from build123d import *

# Parameters (mm, degrees)
SKETCH_1_R          = 1.25
SKETCH_1_R_2        = 1.5
EXTRUDE_1_DEPTH     = 2
CUT_EXTRUDE_1_DEPTH = 10
FILLET_1_R          = 2


with BuildPart() as part:
    # 草图1 → 凸台-拉伸1 (new body)
    with BuildSketch(Plane(origin=(0, 0, 0), x_dir=(1, 0, 0), z_dir=(0, 1, 0))):
        Polygon((11, 0), (-11, 0), (-16.5, -41.3), (-16.5, -120.3), (-16.5, -167.8), (23.75, -167.8), (23.75, -124.8), (16.5, -120.3), (16.5, -41.3), align=None)
        with Locations(Location((-8, -3, 0), (0, 0, 270))):
            Circle(SKETCH_1_R, mode=Mode.SUBTRACT)
        with Locations(Location((-8, -33, 0), (0, 0, 270))):
            Circle(SKETCH_1_R, mode=Mode.SUBTRACT)
        with Locations(Location((8, -33, 0), (0, 0, 90))):
            Circle(SKETCH_1_R, mode=Mode.SUBTRACT)
        with Locations(Location((8, -3, 0), (0, 0, 90))):
            Circle(SKETCH_1_R, mode=Mode.SUBTRACT)
        with Locations(Location((-13, -45.3, 0), (0, 0, 270))):
            Circle(SKETCH_1_R_2, mode=Mode.SUBTRACT)
        with Locations(Location((-13, -105.3, 0), (0, 0, 270))):
            Circle(SKETCH_1_R_2, mode=Mode.SUBTRACT)
        with Locations(Location((-13, -115.3, 0), (0, 0, 270))):
            Circle(SKETCH_1_R_2, mode=Mode.SUBTRACT)
        with Locations(Location((13, -115.3, 0), (0, 0, 90))):
            Circle(SKETCH_1_R_2, mode=Mode.SUBTRACT)
        with Locations(Location((13, -105.3, 0), (0, 0, 90))):
            Circle(SKETCH_1_R_2, mode=Mode.SUBTRACT)
        with Locations(Location((13, -45.3, 0), (0, 0, 90))):
            Circle(SKETCH_1_R_2, mode=Mode.SUBTRACT)
        with Locations(Location((20.75, -129.8, 0), (0, 0, 270))):
            Circle(SKETCH_1_R_2, mode=Mode.SUBTRACT)
        with Locations(Location((20.75, -159.8, 0), (0, 0, 90))):
            Circle(SKETCH_1_R_2, mode=Mode.SUBTRACT)
        with Locations(Location((-9.25, -164.8, 0), (0, 0, 270))):
            Circle(SKETCH_1_R_2, mode=Mode.SUBTRACT)
    extrude(amount=EXTRUDE_1_DEPTH)

    # 草图2 → 切除-拉伸1 (cut)
    with BuildSketch(Plane(origin=(0, 2, 0), x_dir=(1, 0, 0), z_dir=(0, 1, 0))):
        Polygon((6.754889433, -6), (-6.754889433, -6), (-9.951015341, -30), (9.951015341, -30), align=None)
        Polygon((12.5, -97.228932188), (2.5, -87.228932188), (2.5, -39.042640687), (12.5, -49.042640687), align=None)
        Polygon((-12.5, -49.042640687), (-2.5, -39.042640687), (-2.5, -87.228932188), (-12.5, -97.228932188), align=None)
        Polygon((-9.5, -101.3), (0, -91.8), (9.5, -101.3), (9.5, -120.3), (-9.5, -120.3), align=None)
    extrude(amount=-CUT_EXTRUDE_1_DEPTH, mode=Mode.SUBTRACT)

    # 圆角1
    fillet_1_edges = [part.edges().sort_by_distance(p)[0] for p in [
        (-9.951015341, 1, 30),
        (-6.754889433, 1, 6),
        (6.754889433, 1, 6),
        (9.951015341, 1, 30),
        (0, 1, 91.8),
        (9.5, 1, 101.3),
        (9.5, 1, 120.3),
        (-9.5, 1, 120.3),
        (-9.5, 1, 101.3),
        (12.5, 1, 49.042640687),
        (12.5, 1, 97.228932188),
        (2.5, 1, 87.228932188),
        (2.5, 1, 39.042640687),
        (-12.5, 1, 97.228932188),
        (-12.5, 1, 49.042640687),
        (-2.5, 1, 39.042640687),
        (-2.5, 1, 87.228932188),
        (23.75, 1, 124.8),
        (23.75, 1, 167.8),
        (-16.5, 1, 167.8),
        (-11, 1, 0),
        (11, 1, 0),
        (16.5, 1, 120.3),
    ]]
    fillet(fillet_1_edges, radius=FILLET_1_R)


solid = part.part
CAD build for the part. Positions are in the model's coordinates, mm. A direction names the side the tool comes from. Give positions to 0.01 mm unless a question says otherwise; leave off trailing zeros. Loops run counter-clockwise (first coordinate to the right, second up) from the corner with the lowest first, then second, coordinate; pieces in that order, holes last. Notation, with made-up numbers: M 75,-17 L 124,-17 A32 cw 124,15 Z; hole C 9,5 d2. An arc over 180 degrees is marked long. Answer in a Markdown table with one row per item. Add a question column.
Item 1: Probe probe 1 along Z at (x, y) = (-2, 1.15); probe 2 along X at (y, z) = (0.65, 115.3); probe 3 along X at (y, z) = (1.45, 45.3). List the from-to ranges inside material, lowest first.
Item 2: Tool access for faces 4 (the face through (-8.96, 1.01, 45.5)), 5 (the face through (-10, 2, 101)): list every direction of +Z, -Z, +X, -X, +Y, -Y with a clear straight run to the whole face (end or side of a thin tool).
Item 3: Band-saw the part on A-A on z = 129.8. Give the cut face in (x, y), then the cut area to 3 significant figures.
Item 4: Band-saw the part on D-D on z = 45.3. Give the cut face in (x, y), then the cut area to 3 significant figures.
Item 5: Drop a flat-ended pin along its axis: P1, Ø4, axis at x = 20.75, z = 159.8, coming from the +Y side. Give the stop position or say it passes through.
Item 6: Band-saw the part on B-B on z = 78.5. Give the cut face in (x, y).
Item 7: Mould opens along X. For faces 1 (the face through (-5.2, 1, 97)), 2 (the face through (-13.83, 0.99, 21.24)), 3 (the face through (13.9, 0.99, 21.79)) say: +X half, -X half, draft (parallel to the pull), parting line (faces both ways), or undercut.
Item 8: Band-saw the part on C-C on y = 1.05. Give the number of separate pieces and of enclosed holes in the cut face, then the cut area to 3 significant figures.
Reply:
| question | item | result |
|---|---|---|
| 1 | probe 1 | z = 0 to 6, 30 to 93.8, 120.3 to 167.8 |
| 1 | probe 2 | x = -16.5 to -14.5, -11.5 to -9.5, 9.5 to 11.5, 14.5 to 16.5 |
| 1 | probe 3 | x = -16.5 to -14.5, -11.5 to -8.76, -2.5 to 2.5, 8.76 to 11.5, 14.5 to 16.5 |
| 2 | face 4 | +Y, -Y |
| 2 | face 5 | +Z, -Z, +X, -X, +Y |
| 3 | outline | M -16.5,0 L 19.25,0 L 19.25,2 L -16.5,2 Z; M 22.25,0 L 23.75,0 L 23.75,2 L 22.25,2 Z |
| 3 | area | 74.5 mm^2 |
| 4 | outline | M -16.5,0 L -14.5,0 L -14.5,2 L -16.5,2 Z; M -11.5,0 L -8.76,0 L -8.76,2 L -11.5,2 Z; M -2.5,0 L 2.5,0 L 2.5,2 L -2.5,2 Z; M 8.76,0 L 11.5,0 L 11.5,2 L 8.76,2 Z; M 14.5,0 L 16.5,0 L 16.5,2 L 14.5,2 Z |
| 4 | area | 29.0 mm^2 |
| 5 | P1 | stops at y = 2 |
| 6 | outline | M -16.5,0 L -12.5,0 L -12.5,2 L -16.5,2 Z; M -2.5,0 L 2.5,0 L 2.5,2 L -2.5,2 Z; M 12.5,0 L 16.5,0 L 16.5,2 L 12.5,2 Z |
| 7 | face 1 | undercut |
| 7 | face 2 | -X half |
| 7 | face 3 | +X half |
| 8 | separate pieces | 1 |
| 8 | enclosed holes | 17 |
| 8 | area | 3,760 mm^2 |
